Part model, mm, in its own coordinate system. A direction names the side the tool comes from. Round coordinates to 2 decimals unless told otherwise and drop trailing zeros. Write each loop counter-clockwise with the first axis right and the second up, starting at its lowest first coordinate (ties: lowest second). Pieces come first, ordered by that corner, then holes. Notation, with made-up numbers: M 4,11 L 35,11 A10 cw 35,27 Z; hole C -13.5,3.5 d10. An arc over 180 degrees is marked long. Use a Markdown table: item, result. Add a question column.
1) Two-plate mould, pull along X, no slides. Class faces 3 (the face through (27, 3, 17.55)), 4 (the face through (-7.492, 3.288, 11.603)), 5 (the face through (-35, 3, -9)), 6 (the face through (0, 6, 0)): released by +X, released by -X, zero draft, split by the parting line, or undercut.
2) Slice it at D-D on z = -21. Write the cut outline in (x, y), plus the area to 3 significant figures.
3) Which spindle directions (+Z, -Z, +X, -X, +Y, -Y) get a long thin tool onto all of the face, cutting with end or side? Do faces 1 (the face through (30.55, 2.96, -14.94)), 2 (the face through (0, 3, -25)). Say none if no direction does.
4) Slice it at A-A on x = -24. Write the cut outline in (y, z).
5) Slice it at B-B on z = -16. Write the cut outline in (x, y), plus the area to 3 significant figures.
6) Slice it at C-C on y = 1.75. Write the cut outline in (x, z), plus the area to 3 significant figures.
7) Drop flat-ended pins along their axis: P1, Ø5, axis at x = -17.5, z = -16.5, coming from the -Y side; P2, Ø2, axis at x = 27, y = 1.5, coming from the -Z side; P3, Ø0.6, axis at x = 26.5, y = 4, coming from the +Z side. Give the stop position or say it passes through.
8) Wall check: probe 1 along Z at (x, y) = (-25, 3.05); probe 2 along X at (y, z) = (4.1, 13); probe 3 along X at (y, z) = (2.85, -17). Give the ranges that are in metal, low to high.
```python
from build123d import *

# Parameters (mm, degrees)
EXTRUDE_1_DEPTH             = 6
SKETCH_2_R                  = 2.55
CUT_EXTRUDE_1_DEPTH         = 7
CUT_EXTRUDE_2_DEPTH         = 7
HOLE_WIZARD_M52_D           = 5.5
HOLE_WIZARD_M52_CSINK_D     = 11.2
HOLE_WIZARD_M52_CSINK_ANGLE = 90


with BuildPart() as part:
    # Эскиз1 → Бобышка-Вытянуть1 (new body)
    with BuildSketch(Plane(origin=(0, 0, 0), x_dir=(1, 0, 0), z_dir=(0, 1, 0))):
        with BuildLine():
            Line((-25, -25), (25, -25))
            ThreePointArc((25, -25), (32.071067812, -22.071067812), (35, -15))
            Line((35, -15), (35, 15))
            ThreePointArc((35, 15), (32.071067812, 22.071067812), (25, 25))
            Line((25, 25), (-25, 25))
            ThreePointArc((-25, 25), (-32.071067812, 22.071067812), (-35, 15))
            Line((-35, 15), (-35, -15))
            ThreePointArc((-35, -15), (-32.071067812, -22.071067812), (-25, -25))
        make_face()
    extrude(amount=EXTRUDE_1_DEPTH)

    # Эскиз2 → Вырез-Вытянуть1 (cut, through all)
    with BuildSketch(Plane.XZ):
        with Locations((-25, -15)):
            Circle(SKETCH_2_R)
        with Locations((-25, 15)):
            Circle(SKETCH_2_R)
        with BuildLine():
            Line((28, -17.55), (26, -17.55))
            ThreePointArc((26, -17.55), (23.45, -15), (26, -12.45))
            Line((26, -12.45), (28, -12.45))
            ThreePointArc((28, -12.45), (30.55, -15), (28, -17.55))
        make_face()
        with BuildLine():
            Line((28, 17.55), (26, 17.55))
            ThreePointArc((26, 17.55), (23.45, 15), (26, 12.45))
            Line((26, 12.45), (28, 12.45))
            ThreePointArc((28, 12.45), (30.55, 15), (28, 17.55))
        make_face()
    extrude(amount=-CUT_EXTRUDE_1_DEPTH, mode=Mode.SUBTRACT)

    # Эскиз3 → Вырез-Вытянуть2 (cut, through all)
    with BuildSketch(Plane.XZ):
        with BuildLine():
            Line((-35, -2), (-35, 2))
            ThreePointArc((-35, 2), (-34.414213562, 0.585786438), (-33, 0))
            ThreePointArc((-33, 0), (-34.414213562, -0.585786438), (-35, -2))
        make_face()
    extrude(amount=-CUT_EXTRUDE_2_DEPTH, mode=Mode.SUBTRACT)

    # Зенковка для  винта с потайной головкой с внутренним шестигранником M52 (through all)
    with Locations(Plane(origin=(0, 6, 0), x_dir=(1, 0, 0), z_dir=(0, 1, 0))):
        with Locations((-6.159381211, -9.040339254), (-6.159381211, 8.192585184)):
            CounterSinkHole(HOLE_WIZARD_M52_D / 2, HOLE_WIZARD_M52_CSINK_D / 2, counter_sink_angle=HOLE_WIZARD_M52_CSINK_ANGLE)


solid = part.part
```
Entries:
| question | item | result |
|---|---|---|
| 1 | face 3 | undercut |
| 1 | face 4 | undercut |
| 1 | face 5 | released by -X |
| 1 | face 6 | zero draft |
| 2 | outline | M -33,0 L 33,0 L 33,6 L -33,6 Z |
| 2 | area | 396 mm^2 |
| 3 | face 1 | +Y, -Y |
| 3 | face 2 | -Z, +X, -X, +Y, -Y |
| 4 | outline | M 0,-25 L 6,-25 L 6,-17.35 L 0,-17.35 Z; M 0,-12.65 L 6,-12.65 L 6,12.65 L 0,12.65 Z; M 0,17.35 L 6,17.35 L 6,25 L 0,25 Z |
| 5 | outline | M -34.95,0 L -27.35,0 L -27.35,6 L -34.95,6 Z; M -22.65,0 L 23.65,0 L 23.65,6 L -22.65,6 Z; M 30.35,0 L 34.95,0 L 34.95,6 L 30.35,6 Z |
| 5 | area | 351 mm^2 |
| 6 | outline | M -35,-15 A10 ccw -25,-25 L 25,-25 A10 ccw 35,-15 L 35,15 A10 ccw 25,25 L -25,25 A10 ccw -35,15 L -35,2 A2 ccw -33,0 A2 ccw -35,-2 Z; hole C -25,-15 d5.1; hole C -25,15 d5.1; hole C -6.16,-8.19 d5.5; hole C -6.16,9.04 d5.5; hole M 26,-17.55 L 28,-17.55 A2.55 ccw 28,-12.45 L 26,-12.45 A2.55 ccw Z; hole M 26,12.45 L 28,12.45 A2.55 ccw 28,17.55 L 26,17.55 A2.55 ccw Z |
| 6 | area | 3,260 mm^2 |
| 7 | P1 | stops at y = 0 |
| 7 | P2 | stops at z = -24.95 |
| 7 | P3 | stops at z = 24.93 |
| 8 | probe 1 | z = -25 to -17.55, -12.45 to 12.45, 17.55 to 25 |
| 8 | probe 2 | x = -35 to -26.58, -23.42 to 24.42, 29.58 to 35 |
| 8 | probe 3 | x = -34.8 to -26.58, -23.42 to 24.42, 29.58 to 34.8 |
